Here's how the part is built. I have some questions about the finished solid (model axes, mm). Coordinates: 2 decimals unless noted, no trailing zeros. Write each loop counter-clockwise with the first axis right and the second up, starting at its lowest first coordinate (ties: lowest second). Pieces come first, ordered by that corner, then holes. Notation, with made-up numbers: (-24.5, 56) -> (-9.5, 56) arc R16 ccw to (-9.5, 77) -> close; hole circle Ø1 at (-10.75, 31.5). An arc over 180 degrees is marked (long way). Put each result on its own line as item: value.
```python
from build123d import *

# Parameters (mm, degrees)
SKETCH_R        = 12
SKETCH_R_2      = 8
PAD_DEPTH       = 2
CHAMFER_SIZE    = 0.5
CHAMFER001_SIZE = 1


with BuildPart() as part:
    # Sketch → Pad (new body)
    with BuildSketch(Plane.XY):
        Circle(SKETCH_R)
        Circle(SKETCH_R_2, mode=Mode.SUBTRACT)
    extrude(amount=PAD_DEPTH)

    # Chamfer
    chamfer_edges = [part.edges().sort_by_distance(p)[0] for p in [
        (-8, 0, 2),
    ]]
    chamfer(chamfer_edges, length=CHAMFER_SIZE)

    # Chamfer001
    chamfer001_edges = [part.edges().sort_by_distance(p)[0] for p in [
        (-12, 0, 2),
    ]]
    chamfer(chamfer001_edges, length=CHAMFER001_SIZE)


solid = part.part
```
Item 1: Imagine slicing it at A-A on y = 0. Write out the boundary of the cut face in (x, z).
Output:
outline: (-12, 0) -> (-8, 0) -> (-8, 1.5) -> (-8.5, 2) -> (-11, 2) -> (-12, 1) -> close; (8, 0) -> (12, 0) -> (12, 1) -> (11, 2) -> (8.5, 2) -> (8, 1.5) -> close
Item 2: If we mould it in two halves opening along Y, with no side actions, what happens to faces 1 (the cylindrical face through (-11.99, 0.53, 0.49)), 2 (the cylindrical face through (-1.73, -7.81, 0.74)), 3 (the flat face through (2, -8, 0))? For each: released by +Y, released by -Y, zero draft, split by the parting line, or undercut.
Output:
face 1: split by the parting line
face 2: undercut
face 3: zero draft
Item 3: Please list where these lines run through material, in increasing order: line 1 along Y through (x, z) = (0, 0.8); line 2 along Y through (x, z) = (4.5, 1.6); line 3 along X through (y, z) = (6.25, 1.1). Write a range as from..to.
Output:
line 1: y = -12..-8, 8..12
line 2: y = -10.47..-6.73, 6.73..10.47
line 3: x = -10.13..-4.99, 4.99..10.13
